Here's how the part is built. I have some questions about the finished solid (model axes, mm). Face numbers are marked on the shaded views. A direction names the side the tool comes from. Give positions to 0.01 mm unless a question says otherwise; leave off trailing zeros. Write each loop counter-clockwise with the first axis right and the second up, starting at its lowest first coordinate (ties: lowest second). Pieces come first, ordered by that corner, then holes. Notation, with made-up numbers: (-33, -26.75) -> (-16, -26.75) arc R21 cw to (-16, -7.75) -> close; hole circle Ø5 at (66.5, 3.5). An arc over 180 degrees is marked (long way). Use one line per item in the form item = value.
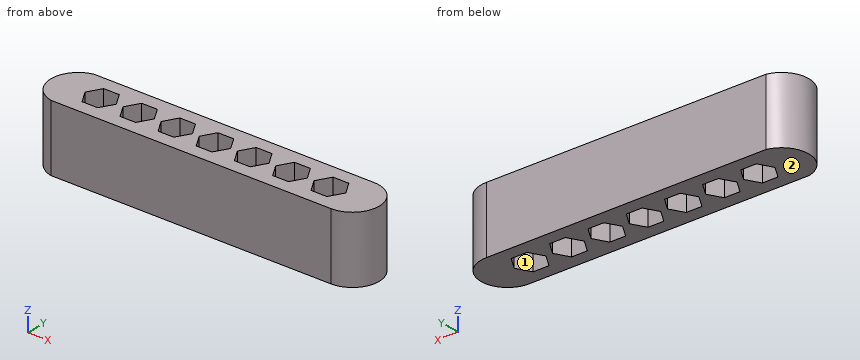
```python
from build123d import *

# Parameters (mm, degrees)
F1_DEPTH = 20


with BuildPart() as f1:
    # F0 (on Top) → F1 (new body)
    with BuildSketch(Plane.XY):
        with BuildLine():
            Line((43.544571, 8.03), (-39.620463, 8.03))
            ThreePointArc((-39.620463, 8.03), (-46.105617, 0), (-39.620463, -8.03))
            Line((-39.620463, -8.03), (43.741562, -8.032416))
            ThreePointArc((43.741562, -8.032416), (51.773374, 0.098503), (43.544571, 8.03))
        make_face()
        Polygon((-26.58473, 0), (-28.911452, -4.03), (-33.564895, -4.03), (-35.891616, 0), (-33.564895, 4.03), (-28.911452, 4.03), align=None, mode=Mode.SUBTRACT)
        Polygon((-22.252235, 4.04), (-17.587245, 4.04), (-15.25475, 0), (-17.587245, -4.04), (-22.252235, -4.04), (-24.58473, 0), align=None, mode=Mode.SUBTRACT)
        Polygon((-13.25475, 0), (-10.916481, 4.05), (-6.239944, 4.05), (-3.901675, 0), (-6.239944, -4.05), (-10.916481, -4.05), align=None, mode=Mode.SUBTRACT)
        Polygon((-1.901675, 0), (0.442367, 4.06), (5.130451, 4.06), (7.474493, 0), (5.130451, -4.06), (0.442367, -4.06), align=None, mode=Mode.SUBTRACT)
        Polygon((9.474493, 0), (11.824309, 4.07), (16.52394, 4.07), (18.873755, 0), (16.52394, -4.07), (11.824309, -4.07), align=None, mode=Mode.SUBTRACT)
        Polygon((20.873755, 0), (23.229345, 4.08), (27.940523, 4.08), (30.296112, 0), (27.940523, -4.08), (23.229345, -4.08), align=None, mode=Mode.SUBTRACT)
        Polygon((32.296112, 0), (34.657474, 4.09), (39.3802, 4.09), (41.741562, 0), (39.3802, -4.09), (34.657474, -4.09), align=None, mode=Mode.SUBTRACT)
    extrude(amount=F1_DEPTH)


solid = f1.part
```
Q1. Will these pins go through, and if not, where does the flat tip stop? pin 1 Ø10 at (x, z) = (-11, 9.5) entering from +Y; pin 2 Ø1.4 at (x, z) = (-31.5, 8.5) entering from -Y.
Result set:
pin_1 = 8.03
pin_2 = -8.03
Q2. I want a section at D-D, the plane x = 2. Write out the boundary of the cut face in (y, z).
Result set:
outline = (-8.03, 0) -> (-4.06, 0) -> (-4.06, 20) -> (-8.03, 20) -> close; (4.06, 0) -> (8.03, 0) -> (8.03, 20) -> (4.06, 20) -> close
Q3. I want a section at A-A, the plane x = 14.5. Write out the boundary of the cut face in (y, z), and give its area (3 significant figures).
Result set:
outline = (-8.03, 0) -> (-4.07, 0) -> (-4.07, 20) -> (-8.03, 20) -> close; (4.07, 0) -> (8.03, 0) -> (8.03, 20) -> (4.07, 20) -> close
area = 158 mm2
Q4. Which directions (+Z, -Z, +X, -X, +Y, -Y) give clear straight access to the entire face, cutting with the end or side of a thin tool? Please do the marked faces 1 and 2.
Result set:
face_1 = +Z, -Z
face_2 = -Z, +X, -X, +Y, -Y
Q5. If I drill on line 1 along Y through (x, z) = (36, 16); line 2 along Y through (x, z) = (-29.5, 1); line 3 along Y through (x, z) = (8, 19), over which ranges is the centre line in solid material (lowest first)? Write a range as from..to.
Result set:
line_1 = -8.03..-4.09, 4.09..8.03
line_2 = -8.03..-4.03, 4.03..8.03
line_3 = -8.03..8.03
Q6. I want a section at B-B, the plane y = -2.75. Count the separate pieces of the cut face and the enclosed holes in it, and give its area (3 significant figures).
Result set:
separate_pieces = 8
enclosed_holes = 0
area = 1,070 mm2
